The listing builds one solid part. Answer for the finished solid, in the listing's coordinates (mm). Face numbers are marked on the shaded views. A direction names the side the tool comes from. Give positions to 0.01 mm unless a question says otherwise; leave off trailing zeros. Loops run counter-clockwise (first coordinate to the right, second up) from the corner with the lowest first, then second, coordinate; pieces in that order, holes last. Notation, with made-up numbers: M -6.75,-30 L 50.25,-30 A13 ccw 50.25,-18 Z; hole C 86,56.5 d11. An arc over 180 degrees is marked long. One line per item, written item: value. Start each with the question number.
Q1. The mould has two halves that part along Y. Classify the marked faces 4, 5 and 6: +Y half, -Y half, draft (parallel to the pull), parting line (faces both ways), or undercut.
Q2. A cutting plane is placed at A-A, the plane y = -9.5. Determine the outline of the cut face in (x, z), and give its area (3 significant figures).
Q3. For the marked faces 1, 2 and 3, determine the directions among +Z, -Z, +X, -X, +Y, -Y from which every point of the face is accessible in a straight line to the end or side of a thin tool.
Q4. Flat-ended cylindrical pins translate along their axes: pin 1 (5 mm diameter, centred on y = 14, z = -3.5, fed in from -X); pin 2 (3.5 mm diameter, centred on y = -4.5, z = 3, fed in from -X); pin 3 (6 mm diameter, centred on x = 10, z = 2.5, fed in from +Y); pin 4 (7.5 mm diameter, centred on x = 0, z = 0, fed in from -Y). Find the tip coordinate at first contact, or state that the pin passes through.
Q5. Consider L1, parallel to X at y = -6.5, z = 0; L2, parallel to Z at x = -5, y = 5.5; L3, parallel to Z at x = 2, y = 8. Determine where each line is inside the solid, lowest interval first.
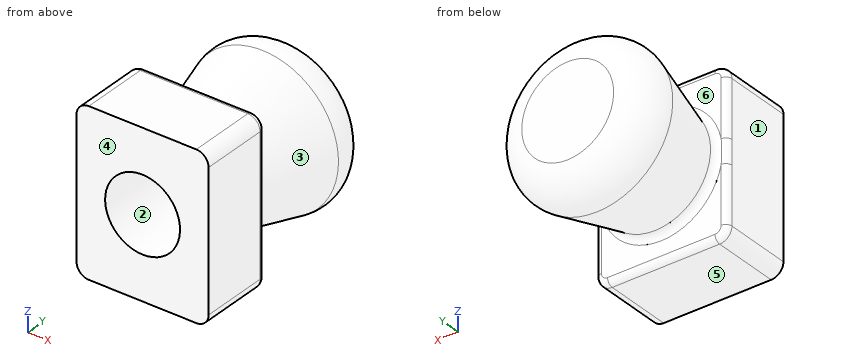
from build123d import *

# Parameters (mm, degrees)
ESQUISSE3_W             = 21.5
ESQUISSE3_H             = 26.5
BOSS_EXTRU_2_DEPTH      = 12
CONG_1_R                = 5
CONG_2_R                = 2
CONG_3_R                = 1
CONG_4_R                = 1
ESQUISSE4_R             = 6.1
ENL_V_MAT_EXTRU_1_DEPTH = 28
CONG_5_R                = 6


with BuildPart() as part:
    # Esquisse2 → Révolution1 (revolve)
    with BuildSketch(Plane.XY, mode=Mode.PRIVATE) as r_volution1_sk:
        Polygon((0, 20), (14, 20), (8.641016151, 0), (0, 0), align=None)
    revolve(r_volution1_sk.sketch.rotate(Axis((0, 0, 0), (0, 1, 0)), 90), axis=Axis((0, 0, 0), (0, 1, 0)))

    # Esquisse3 → Boss.-Extru.2 (add)
    with BuildSketch(Plane.XZ):
        Rectangle(ESQUISSE3_W, ESQUISSE3_H)
    extrude(amount=BOSS_EXTRU_2_DEPTH)

    # Congé1
    cong_1_edges = [part.edges().sort_by_distance(p)[0] for p in [
        (0, 20, 14),
    ]]
    fillet(cong_1_edges, radius=CONG_1_R)

    # Congé2
    cong_2_edges = [part.edges().sort_by_distance(p)[0] for p in [
        (10.75, -6, 13.25),
        (-10.75, -6, 13.25),
        (-10.75, -6, -13.25),
        (10.75, -6, -13.25),
    ]]
    fillet(cong_2_edges, radius=CONG_2_R)

    # Congé3
    cong_3_edges = [part.edges().sort_by_distance(p)[0] for p in [
        (0, 0, 8.641016151),
    ]]
    fillet(cong_3_edges, radius=CONG_3_R)

    # Congé4
    cong_4_edges = [part.edges().sort_by_distance(p)[0] for p in [
        (-10.75, 0, 0),
        (10.75, 0, 0),
        (0, 0, -13.25),
        (0, 0, 13.25),
        (10.164213562, 0, -12.664213562),
        (-10.164213562, 0, -12.664213562),
        (10.164213562, 0, 12.664213562),
        (-10.164213562, 0, 12.664213562),
    ]]
    fillet(cong_4_edges, radius=CONG_4_R)

    # Esquisse4 → Enlèv. mat.-Extru.1 (cut)
    with BuildSketch(Plane.XZ.offset(12)):
        with Locations(Location((0, 0, 0), (0, 0, 270))):
            Circle(ESQUISSE4_R)
    extrude(amount=-ENL_V_MAT_EXTRU_1_DEPTH, mode=Mode.SUBTRACT)

    # Congé5
    cong_5_edges = [part.edges().sort_by_distance(p)[0] for p in [
        (0, 16, 6.1),
    ]]
    fillet(cong_5_edges, radius=CONG_5_R)


solid = part.part
Answer block:
1. face 4: -Y half
1. face 5: draft
1. face 6: undercut
2. outline: M -10.75,-11.25 A2 ccw -8.75,-13.25 L 8.75,-13.25 A2 ccw 10.75,-11.25 L 10.75,11.25 A2 ccw 8.75,13.25 L -8.75,13.25 A2 ccw -10.75,11.25 Z; hole C 0,0 d12.2
2. area: 449 mm^2
3. face 1: +Z, -Z, -X, -Y
3. face 2: -Y
3. face 3: none
4. pin 1: x = -12.43
4. pin 2: x = -10.75
4. pin 3: y = 20
4. pin 4: y = 14.76
5. L1: -10.75 to -6.1, 6.1 to 10.75
5. L2: -8.79 to -3.49, 3.49 to 8.79
5. L3: -10.6 to -5.76, 5.76 to 10.6
